Autodesk Inventor part; units mm, degrees
ref_plane "YZ Plane" through (0, 0, 0) normal (1, 0, 0) x (0, 1, 0)
ref_plane "XZ Plane" through (0, 0, 0) normal (0, 1, 0) x (-1, 0, 0)
ref_plane "XY Plane" through (0, 0, 0) normal (0, 0, 1) x (1, 0, 0)
sketch "Skizze1" plane through (0, 0, 0) normal (0, 1, 0) x (-1, 0, 0)
  line L0 (0, -50) -> (0, -4)
  line L1 (-4, 0) -> (-42, 0)
  line L2 (-42, 0) -> (-42, -3)
  line L3 (-42, -3) -> (-3, -3)
  line L4 (-3, -3) -> (-3, -50)
  line L5 (-3, -50) -> (0, -50)
  arc A0 (0, -4) -> (-4, 0) centre (-4, -4) ccw
  line L6 (0, -60.1657) -> (0, 10.9941)
  line L7 (9.3941, 0) -> (-50.5657, 0)
  point P0 (0, 0)
  point P1 (0, 0)
  dimension "d0" = 42
  dimension "d1" = 50
  dimension "d2" = 3
  dimension "d3" = 4
extrude "Extrusion1" add sketch "Skizze1" along normal mid plane 52 contours L5 L4 L3 L2 L1 A0 L0
fillet "Rundung1" radius 2 4 edges at (1.5, 26, -50) (1.5, -26, -50) (42, 26, -1.5) (42, -26, -1.5)
sketch "Skizze2" plane through (4, -26, 0) normal (0, 0, 1) x (1, 0, 0)
  circle A0 centre (5, 28) radius 2.5
  circle A1 centre (30, 28) radius 2.5
  line L0 (38, 2) -> (38, 50)
  line L1 (-166, 18) -> (204, 18)
  line L2 (-1, 0) -> (36, 0)
  line L3 (204, 18) -> (-166, 18)
  point P0 (-4, 26)
  point P1 (38, 26)
  dimension "d7" = 5
  dimension "d8" = 8
  dimension "d9" = 25
  dimension "d25" = 10
  dimension "d26" = 10
extrude "Extrusion2" cut sketch "Skizze2" against normal through all
sketch "Skizze3" plane through (0, -26, -4) normal (-1, 0, 0) x (0, 0, 1)
  circle A0 centre (-40.5, 43.5) radius 1.5
  circle A1 centre (-9.5, 43.5) radius 1.5
  circle A2 centre (-9.5, 12.5) radius 1.5
  circle A3 centre (-40.5, 12.5) radius 1.5
  circle A4 centre (-25, 28) radius 10
  line L0 (-46, 50) -> (-46, 2)
  line L1 (-25, 41.9808) -> (-25, 15.4808)
  circle A5 centre (-25, 28) radius 2.5
  point P0 (4, 26)
  dimension "d12" = 31
  dimension "d13" = 31
  dimension "d14" = 3
  dimension "d16" = 20
  dimension "d21" = 15.5
  dimension "d22" = 31
extrude "Extrusion3" cut sketch "Skizze3" against normal through all
properties part number "YAufnahmeMotor"
Can you work these out from the model? Positions are in its coordinate system, mm. A direction names the side the tool comes from. Give positions to 0.01 mm unless a question says otherwise; leave off trailing zeros. Order: outer loops, then holes, each group sorted by start corner. A loop starts at its lowest first (then second) coordinate and runs counter-clockwise, first axis right, second up. Notation, with made-up numbers: (-9, 88) - (38, 88) arc R16 cw to (38, 112) - close; hole circle Ø11 at (54.25, 63.25). An arc over 180 degrees is marked (long way). Use a Markdown table: item, result. Add a question column.
Q1. If we section it at C-C on x = 9: Write out the boundary of the cut face in (y, z), plus the area to 3 significant figures.
Q2. Please list where these lines run through material, in increasing order: line 1 along Y through (x, z) = (2.1, -13.5); line 2 along Y through (x, z) = (2, -29); line 3 along Y through (x, z) = (2.5, -14.5).
Q3. If we section it at B-B on y = 2: Write out the boundary of the cut face in (x, z), plus the area to 3 significant figures.
Q4. I'm going to push flat-ended pins straight in: pin 1 (12 mm diameter, centred on y = 2, z = -29, fed in from -X); pin 2 (19.5 mm diameter, centred on x = 16.5, y = 8.5, fed in from -Z); pin 3 (4 mm diameter, centred on x = 5, y = -6.5, fed in from +Z); pin 4 (1 mm diameter, centred on y = 13.5, z = -25, fed in from +X). Where does each tip first touch, or does it pass through?
Q5. On a 3-axis mill with a long thin cutter (end or side, diameter ignored), from which of +Z, -Z, +X, -X, +Y, -Y can I reach the whole of each face in a straight line? I mean faces 1 (the flat face through (23, 0, -3)), 2 (the cylindrical face through (8.46, -0.44, -1.48)). Say none if no direction works.
Q6. If we section it at A-A on z = -29: Write out the boundary of the cut face in (x, y), plus the area to 3 significant figures.
Q7. If we mould it in two halves opening along Z, with no side actions, what happens to faces 3 (the cylindrical face through (1.48, 5, -19.46)), 4 (the cylindrical face through (1.48, 25.43, -49.4)), 5 (the flat face through (2, 26, -13))? For each: released by +Z, released by -Z, zero draft, split by the parting line, or undercut.
Q8. If we section it at D-D on z = -13.5: Write out the boundary of the cut face in (x, y), plus the area to 3 significant figures.
Answers follow:
| question | item | result |
|---|---|---|
| 1 | outline | (-26, -3) - (-0.5, -3) - (-0.5, 0) - (-26, 0) - close; (4.5, -3) - (26, -3) - (26, 0) - (4.5, 0) - close |
| 1 | area | 141 mm^2 |
| 2 | line 1 | y = -26 to -15, -12 to 16, 19 to 26 |
| 2 | line 2 | y = -26 to -8, 12 to 26 |
| 2 | line 3 | y = -26 to -14.62, -12.38 to 16.38, 18.62 to 26 |
| 3 | outline | (0, -50) - (3, -50) - (3, -39) - (0, -39) - close; (0, -19) - (3, -19) - (3, -3) - (6.5, -3) - (6.5, 0) - (4, 0) arc R4 ccw to (0, -4) - close; (11.5, -3) - (31.5, -3) - (31.5, 0) - (11.5, 0) - close; (36.5, -3) - (42, -3) - (42, 0) - (36.5, 0) - close |
| 3 | area | 174 mm^2 |
| 4 | pin 1 | passes through |
| 4 | pin 2 | stops at z = -3 |
| 4 | pin 3 | stops at z = 0 |
| 4 | pin 4 | stops at x = 3 |
| 5 | face 1 | -Z, +X, +Y, -Y |
| 5 | face 2 | +Z, -Z |
| 6 | outline | (0, -26) - (3, -26) - (3, -8) - (0, -8) - close; (0, 12) - (3, 12) - (3, 26) - (0, 26) - close |
| 6 | area | 96.0 mm^2 |
| 7 | face 3 | undercut |
| 7 | face 4 | released by -Z |
| 7 | face 5 | zero draft |
| 8 | outline | (0, -26) - (3, -26) - (3, -15) - (0, -15) - close; (0, -12) - (3, -12) - (3, 16) - (0, 16) - close; (0, 19) - (3, 19) - (3, 26) - (0, 26) - close |
| 8 | area | 138 mm^2 |
